Build history of the part. All positions in model axes, mm. A direction names the side the tool comes from. Coordinates: 2 decimals unless noted, no trailing zeros. Write each loop counter-clockwise with the first axis right and the second up, starting at its lowest first coordinate (ties: lowest second). Pieces come first, ordered by that corner, then holes. Notation, with made-up numbers: (-32, 47) -> (-19, 47) arc R18 ccw to (-19, 71) -> close; hole circle Ø10 at (28, -28). An arc over 180 degrees is marked (long way). Write each question's results on one line, items separated by ' | '. Start each with the question number.
Q1. Saw through at B-B on y = 2.35. Count the separate pieces of the cut face and the enclosed holes in it, and give its area (3 significant figures).
Q2. Saw through at A-A on x = 78.5. Give the cut face in (y, z) (3 decimals), and give its area (3 significant figures).
Q3. Drop flat-ended pins along their axis: pin 1 Ø1 at (y, z) = (1.5, 10) entering from -X; pin 2 Ø1.5 at (y, z) = (1.5, -38.5) entering from -X. Give the stop position or say it passes through.
Q4. Tool access for faces 4 (the face through (3, 3.175, -33)), 5 (the face through (-32.31, 1.61, -54.67)): list every direction of +Z, -Z, +X, -X, +Y, -Y with a clear straight run to the whole face (end or side of a thin tool).
Q5. Two-plate mould, pull along X, no slides. Class faces 1 (the face through (3.1, 1.57, 158.72)), 2 (the face through (17.29, 1.57, 127.74)), 3 (the face through (3, 0, -33)): released by +X, released by -X, zero draft, split by the parting line, or undercut.
Q6. Drill centre lines: line 1 (Z direction, x = -28, y = 1.85); line 2 (X direction, y = 1.9, z = 13.5); line 3 (X direction, y = 0.8, z = 15). Where is each one in solid material? Low to high.
Autodesk Inventor part; units mm, degrees
ref_plane "YZ Plane" through (0, 0, 0) normal (1, 0, 0) x (0, 1, 0)
ref_plane "XZ Plane" through (0, 0, 0) normal (0, 1, 0) x (-1, 0, 0)
ref_plane "XY Plane" through (0, 0, 0) normal (0, 0, 1) x (1, 0, 0)
sketch "Sketch1" plane through (0, 0, 0) normal (0, 1, 0) x (-1, 0, 0)
  circle A0 centre (0, 0) radius 158.75
  line L0 (26.05, 30.05) -> (-26.05, 30.05)
  line L1 (-30.05, 26.05) -> (-30.05, -26.05)
  line L2 (-26.05, -30.05) -> (26.05, -30.05)
  line L3 (30.05, -26.05) -> (30.05, 26.05)
  arc A1 (30.05, 26.05) -> (26.05, 30.05) centre (26.05, 26.05) ccw
  arc A2 (26.05, -30.05) -> (30.05, -26.05) centre (26.05, -26.05) ccw
  arc A3 (-30.05, -26.05) -> (-26.05, -30.05) centre (-26.05, -26.05) ccw
  arc A4 (-26.05, 30.05) -> (-30.05, 26.05) centre (-26.05, 26.05) ccw
  circle A5 centre (38, 0) radius 2.5527
  circle A6 centre (0, -38) radius 2.5527
  circle A7 centre (-38, 0) radius 2.5527
  circle A8 centre (0, 38) radius 2.5527
  circle A9 centre (63.9092, 0) radius 4.7625
  circle A10 centre (-31.9546, -55.3454) radius 4.7625
  circle A11 centre (0, 0) radius 63.9092 construction
  circle A12 centre (0, 143.6497) radius 3.2067
  circle A13 centre (0, -143.6497) radius 3.2067
  line L4 (157.6029, 19.05) -> (165.227, 19.05)
  line L5 (165.227, 19.05) -> (165.227, -19.05) construction
  line L6 (165.227, -19.05) -> (157.6029, -19.05)
  line L7 (157.6029, -17.4578) -> (157.6029, 19.05) construction
  arc A14 (165.227, -19.05) -> (165.227, 19.05) centre (165.227, 0) ccw
  circle A15 centre (165.227, 0) radius 3.2067
  line L8 (0, -158.75) -> (0, 158.75) construction
  line L9 (-157.6029, 19.05) -> (-165.227, 19.05)
  line L10 (-165.227, -19.05) -> (-157.6029, -19.05)
  arc A16 (-165.227, 19.05) -> (-165.227, -19.05) centre (-165.227, 0) ccw
  circle A17 centre (-165.227, 0) radius 3.2067
  circle A18 centre (-31.9533, 55.3478) radius 4.7625
  point P0 (30.05, 30.05)
  point P1 (-30.05, 30.05)
  point P2 (30.05, -30.05)
  dimension "d0" = 317.5
  dimension "d1" = 30.05
  dimension "d2" = 60.1
  dimension "d3" = 60.1
  dimension "d4" = 30.05
  dimension "d5" = 4
  dimension "d6" = 4
  dimension "d7" = 5.1054
  dimension "d8" = 5.1054
  dimension "d9" = 5.1054
  dimension "d10" = 5.1054
  dimension "d11" = 76
  dimension "d12" = 38
  dimension "d13" = 76
  dimension "d14" = 38
  dimension "d15" = 9.525
  dimension "d17" = 110.6932
  dimension "d20" = 9.525
  dimension "d24" = 6.4135
  dimension "d25" = 6.4135
  dimension "d26" = 287.2994
  dimension "d27" = 143.6497
  dimension "d30" = 38.1
  dimension "d31" = 6.4135
  dimension "d33" = 330.454
  dimension "d38" = 110.6932
  dimension "d39" = 110.6932
  dimension "d41" = 127.8184
extrude "Extrusion1" add sketch "Sketch1" along normal blind 3.175
fillet "Fillet1" radius 10.16 4 edges at (-157.6029, 1.5875, 19.05) (-157.6029, 1.5875, -19.05) (157.6029, 1.5875, -19.05) (157.6029, 1.5875, 19.05)
sketch "Sketch2" plane through (0, 3.175, 0) normal (0, 1, 0) x (1, 0, 0)
  line L0 (63.5, 50.8) -> (102.4151, 83.4536)
  line L1 (63.5, 50.8) -> (63.5, -50.8)
  line L2 (63.5, -50.8) -> (102.4151, -83.4536)
  arc A0 (102.4151, -83.4536) -> (102.4151, 83.4536) centre (0, 0) ccw
  line L3 (-75.7441, 29.5926) -> (-123.4805, 46.9672)
  line L4 (12.2441, 80.3926) -> (21.0654, 130.4208)
  line L5 (-75.7441, 29.5926) -> (12.2441, 80.3926)
  arc A1 (21.0654, 130.4208) -> (-123.4805, 46.9672) centre (0, 0) ccw
  line L6 (12.2441, -80.3926) -> (21.0654, -130.4208)
  line L7 (-75.7441, -29.5926) -> (-123.4805, -46.9672)
  line L8 (12.2441, -80.3926) -> (-75.7441, -29.5926)
  arc A2 (-123.4805, -46.9672) -> (21.0654, -130.4208) centre (0, 0) ccw
  point P0 (0, 0)
  dimension "d42" = 101.6
  dimension "d43" = 50.8
  dimension "d44" = 130
  dimension "d45" = 130
  dimension "d46" = 50.8
  dimension "d47" = 50.8
  dimension "d48" = 63.5
  dimension "d49" = 0
  dimension "d52" = 360
extrude "Extrusion2" cut sketch "Sketch2" against normal blind 6.35
fillet "Fillet2" radius 10.16 6 edges at (-123.4805, 1.5875, 46.9672) (21.0654, 1.5875, -130.4208) (102.4151, 1.5875, -83.4536) (21.0654, 1.5875, 130.4208) (102.4151, 1.5875, 83.4536) (-123.4805, 1.5875, -46.9672)
fillet "Fillet3" radius 10.16 6 edges at (-75.7441, 1.5875, -29.5926) (63.5, 1.5875, -50.8) (12.2441, 1.5875, 80.3926) (-75.7441, 1.5875, 29.5926) (63.5, 1.5875, 50.8) (12.2441, 1.5875, -80.3926)
sketch "Sketch3" plane through (0, 3.175, 0) normal (0, 1, 0) x (1, 0, 0)
  arc A0 (156.3619, 27.432) -> (-156.3619, 27.432) centre (0, 0) ccw
  line L0 (82.2664, 135.7711) -> (76.6274, 126.5262)
  line L1 (71.6492, 125.9572) -> (67.3261, 130.3685)
  line L2 (62.348, 129.7996) -> (52.2012, 113.1643)
  line L3 (54.9118, 108.336) -> (59.8766, 108.336)
  line L4 (62.5872, 103.5077) -> (59.6212, 98.6449)
  line L5 (62.1502, 93.8218) -> (68.5548, 93.4551)
  line L6 (70.903, 88.3667) -> (56.7738, 69.7364)
  line L7 (51.3067, 70.4499) -> (48.2668, 77.8597)
  line L8 (43.6958, 79.3771) -> (21.3897, 65.9934)
  line L9 (19.9367, 64.015) -> (15.5672, 45.89)
  line L10 (18.312, 41.9894) -> (42.8589, 39.3314)
  line L11 (45.5063, 35.1047) -> (41.1925, 23.0559)
  line L12 (39.4084, 21.1887) -> (30.05, 17.3494)
  line L13 (30.05, 26.05) -> (30.05, -26.05)
  arc A1 (71.6492, 125.9572) -> (76.6274, 126.5262) centre (73.9169, 128.1795) ccw
  arc A2 (67.3261, 130.3685) -> (62.348, 129.7996) centre (65.0585, 128.1462) ccw
  arc A3 (52.2012, 113.1643) -> (54.9118, 108.336) centre (54.9118, 111.511) ccw
  arc A4 (70.903, 88.3667) -> (68.5548, 93.4551) centre (68.3733, 90.2853) ccw
  arc A5 (62.5872, 103.5077) -> (59.8766, 108.336) centre (59.8766, 105.161) ccw
  arc A6 (51.3067, 70.4499) -> (56.7738, 69.7364) centre (54.2441, 71.655) ccw
  arc A7 (48.2668, 77.8597) -> (43.6958, 79.3771) centre (45.3294, 76.6546) ccw
  arc A8 (21.3897, 65.9934) -> (19.9367, 64.015) centre (23.0232, 63.2709) ccw
  arc A9 (15.5672, 45.89) -> (18.312, 41.9894) centre (18.6538, 45.1459) ccw
  arc A10 (45.5063, 35.1047) -> (42.8589, 39.3314) centre (42.5171, 36.1749) ccw
  arc A11 (39.4084, 21.1887) -> (41.1925, 23.0559) centre (38.2034, 24.1261) ccw
  arc A12 (59.6212, 98.6449) -> (62.1502, 93.8218) centre (62.3317, 96.9916) ccw
  line L14 (-157.7126, 3.3351) -> (-147.8886, 3.0982)
  line L15 (-144.9068, -0.9286) -> (-146.5655, -6.8781)
  line L16 (-143.5837, -10.9049) -> (-124.1038, -11.3746)
  line L17 (-121.2776, -6.613) -> (-123.76, -2.3133)
  arc A13 (-120.9339, 2.4483) -> (-123.76, -2.3133) centre (-121.0104, -0.7258) ccw
  arc A14 (-124.1038, -11.3746) -> (-121.2776, -6.613) centre (-124.0272, -8.2005) ccw
  arc A15 (-144.9068, -0.9286) -> (-147.8886, 3.0982) centre (-147.9651, -0.0759) ccw
  arc A16 (-146.5655, -6.8781) -> (-143.5837, -10.9049) centre (-143.5072, -7.7308) ccw
  line L18 (-120.9339, 2.4483) -> (-115.2396, 2.311)
  line L19 (-112.3272, 6.9128) -> (-115.2119, 12.6427)
  line L20 (-111.9793, 17.2205) -> (-88.7805, 14.2994)
  line L21 (-86.6648, 9.2079) -> (-91.5618, 2.8704)
  arc A17 (-111.9793, 17.2205) -> (-115.2119, 12.6427) centre (-112.376, 14.0704) ccw
  arc A18 (-115.2396, 2.311) -> (-112.3272, 6.9128) centre (-115.1631, 5.4851) ccw
  arc A19 (-91.5618, 2.8704) -> (-90.5905, -1.8469) centre (-89.0495, 0.9291) ccw
  arc A20 (-86.6648, 9.2079) -> (-88.7805, 14.2994) centre (-89.1771, 11.1492) ccw
  line L22 (-90.5905, -1.8469) -> (-67.8469, -14.4727)
  line L23 (-65.4069, -14.7418) -> (-47.5255, -9.4634)
  line L24 (-45.5199, -5.136) -> (-55.4915, 17.4512)
  line L25 (-53.1547, 21.8573) -> (-40.5633, 24.1458)
  line L26 (-38.0542, 23.5343) -> (-30.05, 17.3494)
  arc A21 (-67.8469, -14.4727) -> (-65.4069, -14.7418) centre (-66.3058, -11.6967) ccw
  arc A22 (-53.1547, 21.8573) -> (-55.4915, 17.4512) centre (-52.5869, 18.7334) ccw
  arc A23 (-47.5255, -9.4634) -> (-45.5199, -5.136) centre (-48.4244, -6.4183) ccw
  arc A24 (-38.0542, 23.5343) -> (-40.5633, 24.1458) centre (-39.9955, 21.022) ccw
  line L27 (76.448, -139.1304) -> (71.2612, -129.6244)
  line L28 (73.2575, -125.0287) -> (79.2394, -123.4904)
  line L29 (81.2357, -118.8947) -> (71.9026, -101.7897)
  line L30 (66.3658, -101.723) -> (63.8834, -106.0227)
  arc A25 (58.3467, -105.9559) -> (63.8834, -106.0227) centre (61.1338, -104.4352) ccw
  arc A26 (71.9026, -101.7897) -> (66.3658, -101.723) centre (69.1155, -103.3105) ccw
  arc A27 (73.2575, -125.0287) -> (71.2612, -129.6244) centre (74.0483, -128.1036) ccw
  arc A28 (79.2394, -123.4904) -> (81.2357, -118.8947) centre (78.4486, -120.4155) ccw
  line L31 (58.3467, -105.9559) -> (55.6184, -100.9559)
  line L32 (50.177, -100.7346) -> (46.6571, -106.0977)
  line L33 (41.0763, -105.5872) -> (32.0066, -84.0358)
  line L34 (35.3581, -79.6578) -> (43.2951, -80.7301)
  arc A29 (41.0763, -105.5872) -> (46.6571, -106.0977) centre (44.0027, -104.3556) ccw
  arc A30 (55.6184, -100.9559) -> (50.177, -100.7346) centre (52.8313, -102.4767) ccw
  arc A31 (43.2951, -80.7301) -> (46.8947, -77.5303) centre (43.7201, -77.5837) ccw
  arc A32 (35.3581, -79.6578) -> (32.0066, -84.0358) centre (34.933, -82.8043) ccw
  line L35 (46.8947, -77.5303) -> (46.4571, -51.5208)
  line L36 (45.4703, -49.2732) -> (31.9583, -36.4266)
  line L37 (27.2079, -36.8534) -> (12.6326, -56.7826)
  line L38 (7.6484, -56.9619) -> (-0.6292, -47.2018)
  line L39 (-1.3542, -44.7231) -> (0, -34.6988)
  arc A33 (46.4571, -51.5208) -> (45.4703, -49.2732) centre (43.2826, -51.5742) ccw
  arc A34 (7.6484, -56.9619) -> (12.6326, -56.7826) centre (10.0698, -54.9083) ccw
  arc A35 (31.9583, -36.4266) -> (27.2079, -36.8534) centre (29.7706, -38.7277) ccw
  arc A36 (-1.3542, -44.7231) -> (-0.6292, -47.2018) centre (1.7922, -45.1481) ccw
  line L40 (-30.05, -26.05) -> (-30.05, 26.05)
  line L41 (0, -34.6988) -> (0.628, -30.05)
  line L42 (26.05, -30.05) -> (-26.05, -30.05)
  line L43 (-159.5209, 3.9541) -> (-175.7168, 15.9018)
  arc A37 (-165.9718, 19.0354) -> (-165.9718, -19.0354) centre (-165.227, 0) ccw
  arc A38 (-159.5209, 3.9541) -> (-157.7126, 3.3351) centre (-157.6361, 6.5092) ccw
  point P0 (65.5323, 108.336)
  point P1 (56.8639, 94.1245)
  point P2 (-158.7145, 3.3592)
  point P3 (-126.5879, 2.5846)
  point P4 (-109.9462, 2.1833)
  point P5 (61.0556, -110.9206)
  point P6 (53.0823, -96.3078)
  dimension "d58" = 3.175
  dimension "d61" = 360
  dimension "d63" = 3.175
split "Split5" [suppressed]
split "Split8" [suppressed]
split "Split9" [suppressed]
combine "Combine1" [suppressed]
feature "Move Body1" [suppressed]
feature "Move Body2" [suppressed]
feature "Move Body3" [suppressed]
feature "Move Body4" [suppressed]
feature "Move Body5" [suppressed]
equation "\"d24\" = d25"
equation "\"d25\" = d31"
equation "\"d38\" = d17"
equation "\"d39\" = d17"
Returned:
1) separate pieces: 1 | enclosed holes: 15 | area: 51,200 mm2
2) outline: (0, -137.983) -> (3.175, -137.983) -> (3.175, -63.386) -> (0, -63.386) -> close; (0, 63.386) -> (3.175, 63.386) -> (3.175, 137.983) -> (0, 137.983) -> close | area: 474 mm2
3) pin 1: stops at x = -181.74 | pin 2: stops at x = -154.2
4) face 4: +Z, -Z, +X, -X, +Y | face 5: +Y, -Y
5) face 1: split by the parting line | face 2: undercut | face 3: zero draft
6) line 1: z = -156.26 to -129.11, -57.16 to -29.54, 29.54 to 57.16, 129.11 to 156.26 | line 2: x = -178.67 to -30.05, 30.05 to 63.5, 131.42 to 178.67 | line 3: x = -176.97 to -30.05, 30.05 to 63.5, 131.26 to 176.97
